Source: CAD feature listing. Evaluate the final solid. Frame: model axes, mm. Face numbers are marked on the shaded views. Round coordinates to 2 decimals unless told otherwise and drop trailing zeros. Loops run counter-clockwise (first coordinate to the right, second up) from the corner with the lowest first, then second, coordinate; pieces in that order, holes last.
(1) Section B-B, the plane x = 0. Return the cut outline in (y, z).
(2) Section C-C, the plane y = -7. Return the cut outline in (x, z), plus the area to 3 significant figures.
(3) Material intervals for probe 1 along X at (y, z) = (-7.9, 0); probe 2 along Y at (x, z) = (30, 44.5), sorted ascending.
(4) Section A-A, the plane z = 0. Return the cut outline in (x, y), plus the area to 3 significant figures.
(5) Mould query, pull axis X, two halves, no side actions, for the marked faces 1 and 2. Classes: pulls with the +X half, pulls with the -X half, needs draft (parallel to the pull), parting line crosses it, or undercut.
(6) First-contact query: pin 1 Ø3 at (y, z) = (-3.5, -46.5) entering from +X; pin 2 Ø2 at (x, y) = (-8, -2) entering from +Z; pin 3 Ø4 at (x, z) = (21, 29.5) entering from -Y. Flat tips, straight axial feed; report the tip coordinate or a pass-through.
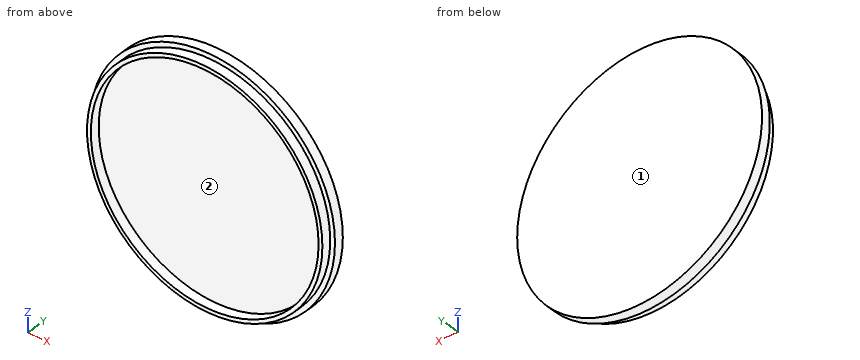
```python
from build123d import *

# Parameters (mm, degrees)
F0_R     = 64.5
F0_R_2   = 62
F0_R_3   = 60
F1_DEPTH = 5
F2_DEPTH = 10


with BuildPart() as f1:
    # F0 (on Front) → F1 (new body)
    with BuildSketch(Plane.XZ):
        Circle(F0_R)
        Circle(F0_R_2, mode=Mode.SUBTRACT)
        Circle(F0_R_2)
        Circle(F0_R_3, mode=Mode.SUBTRACT)
        Circle(F0_R_3)
    extrude(amount=F1_DEPTH)

    # F0 (on Front) → F2 (join)
    with BuildSketch(Plane.XZ):
        Circle(F0_R_2)
        Circle(F0_R_3, mode=Mode.SUBTRACT)
    extrude(amount=F2_DEPTH)


solid = f1.part
```
Output values:
1. outline: (-10, -62) - (-5, -62) - (-5, -64.5) - (0, -64.5) - (0, 64.5) - (-5, 64.5) - (-5, 62) - (-10, 62) - (-10, 60) - (-5, 60) - (-5, -60) - (-10, -60) - close
2. outline: circle Ø124 at (0, 0); hole circle Ø120 at (0, 0)
2. area: 767 mm2
3. probe 1: x = -62 to -60, 60 to 62
3. probe 2: y = -5 to 0
4. outline: (-64.5, -5) - (-62, -5) - (-62, -10) - (-60, -10) - (-60, -5) - (60, -5) - (60, -10) - (62, -10) - (62, -5) - (64.5, -5) - (64.5, 0) - (-64.5, 0) - close
4. area: 665 mm2
5. face 1: needs draft
5. face 2: undercut
6. pin 1: stops at x = 46.21
6. pin 2: stops at z = 64.12
6. pin 3: stops at y = -5
